```python
from build123d import *

# Parameters (mm, degrees)
SKETCH1_W                      = 19.05
SKETCH1_H                      = 57.15
BOSS_EXTRUDE1_DEPTH            = 25.4
SKETCH8_R                      = 65.0875
CUT_EXTRUDE2_DEPTH             = 89.102674477
SKETCH2_W                      = 17.4625
SKETCH2_H                      = 19.05
SKETCH2_W_2                    = 9.525
CUT_EXTRUDE1_DEPTH             = 43.715256349
CBORE_FOR_M4_SHCS1_D           = 4.5
CBORE_FOR_M4_SHCS1_CBORE_D     = 8
CBORE_FOR_M4_SHCS1_CBORE_DEPTH = 4
SKETCH9_R                      = 3.175
CUT_EXTRUDE3_DEPTH             = 93.307357677
CUT_EXTRUDE4_START             = -6.35
CUT_EXTRUDE4_DEPTH             = 25.4
FILLET1_R                      = 6.35
FILLET2_R                      = 6.35


# Read off the part's stored shape, not the designer's step: Cut-Extrude4
with BuildPart() as part:
    # Sketch1 → Boss-Extrude1 (new body)
    with BuildSketch(Plane(origin=(0, 0, 0), x_dir=(1, 0, 0), z_dir=(0, 1, 0))):
        with Locations((69.85, 0)):
            Rectangle(SKETCH1_W, SKETCH1_H)
    extrude(amount=BOSS_EXTRUDE1_DEPTH)

    # Sketch8 → Cut-Extrude2 (cut, through all)
    with BuildSketch(Plane(origin=(0, 25.4, 0), x_dir=(1, 0, 0), z_dir=(0, 1, 0))):
        Circle(SKETCH8_R)
    extrude(amount=-CUT_EXTRUDE2_DEPTH, mode=Mode.SUBTRACT)

    # Sketch2 → Cut-Extrude1 (cut, through all)
    with BuildSketch(Plane(origin=(79.375, 0, 0), x_dir=(0, 0, -1), z_dir=(1, 0, 0))):
        with Locations((-19.84375, 15.875)):
            Rectangle(SKETCH2_W, SKETCH2_H)
        with Locations((0, 15.875)):
            Rectangle(SKETCH2_W_2, SKETCH2_H)
        with Locations((19.84375, 15.875)):
            Rectangle(SKETCH2_W, SKETCH2_H)
    extrude(amount=-CUT_EXTRUDE1_DEPTH, mode=Mode.SUBTRACT)

    # CBORE for M4 SHCS1 (through all)
    with Locations(Plane(origin=(0, 6.35, 0), x_dir=(1, 0, 0), z_dir=(0, 1, 0))):
        with Locations((69.923370565, -18.735910675), (69.923370565, 18.735910675)):
            CounterBoreHole(CBORE_FOR_M4_SHCS1_D / 2, CBORE_FOR_M4_SHCS1_CBORE_D / 2, CBORE_FOR_M4_SHCS1_CBORE_DEPTH)

    # Sketch9 → Cut-Extrude3 (cut, through all)
    with BuildSketch(Plane.XY.offset(11.1125)):
        with Locations(Location((71.753428179, 19.05, 0), (0, 0, 90))):
            Circle(SKETCH9_R)
    extrude(amount=-CUT_EXTRUDE3_DEPTH, mode=Mode.SUBTRACT)

    # Cut-Extrude4 outline → Cut-Extrude4 (cut)
    with BuildSketch(Plane(origin=(0, 6.35, 0), x_dir=(1, 0, 0), z_dir=(0, 1, 0)).offset(CUT_EXTRUDE4_START)):
        with BuildLine():
            ThreePointArc((74.053089065, 28.575), (78.033180665, 14.533180665), (79.375, 0))
            Line((79.375, 0), (79.375, 28.575))
            Line((79.375, 28.575), (74.053089065, 28.575))
        make_face()
        with BuildLine():
            ThreePointArc((79.375, 0), (78.033180665, -14.533180665), (74.053089065, -28.575))
            Line((74.053089065, -28.575), (79.375, -28.575))
            Line((79.375, -28.575), (79.375, 0))
        make_face()
    extrude(amount=CUT_EXTRUDE4_DEPTH, mode=Mode.SUBTRACT)

    # Fillet1
    fillet1_edges = [part.edges().sort_by_distance(p)[0] for p in [
        (78.976482118, 25.4, 7.943922032),
        (78.976482118, 25.4, -7.943922032),
        (64.600512324, 25.4, 7.947104106),
        (64.600512324, 25.4, -7.947104106),
    ]]
    fillet(fillet1_edges, radius=FILLET1_R)

    # Fillet2
    # the kernel refuses this fillet: 6.35 mm, written as the material it takes off along each edge
    with BuildSketch(Plane(origin=(60.325, -14.878589634, -28.575), x_dir=(1, 0, 0), z_dir=(0, 1, 0))) as fillet2_piece_1:
        with BuildLine():
            CenterArc((5.951435854, -6.35), FILLET2_R, 90, 69.592112093)
            Line((0, -4.135748145), (-0.119028717, -4.091463108))
            ThreePointArc((-0.119028717, -4.091463108), (-0.127, -2.067874072), (-0.127, 0))
            Line((-0.127, 0), (0, 0.127))
            Line((0, 0.127), (5.951435854, 0.127))
            Line((5.951435854, 0.127), (5.951435854, 0))
        make_face()
    extrude(amount=36.107179269, mode=Mode.SUBTRACT)
    with BuildSketch(Plane(origin=(74.053089065, -11.708929515, -28.575), x_dir=(0.33231857215714583, 0, 0.9431671997050343), z_dir=(0, 1, 0))) as fillet2_piece_2:
        with BuildLine():
            CenterArc((4.496228934, -6.347235827), FILLET2_R, 88.309367925, 72.281068131)
            Line((-1.492882784, -4.237012894), (-1.612665019, -4.194808436))
            Line((-1.612665019, -4.194808436), (-0.119782234, 0.042204459))
            Line((-0.119782234, 0.042204459), (-0.003746857, 0.126944717))
            ThreePointArc((-0.003746857, 0.126944717), (2.341785903, 0.161552158), (4.687318663, 0.126944717))
            Line((4.687318663, 0.126944717), (4.683571806, 0))
        make_face()
    extrude(amount=29.76785903, mode=Mode.SUBTRACT)
    with BuildSketch(Plane(origin=(60.325, -14.878589634, 28.575), x_dir=(1, 0, 0), z_dir=(0, 1, 0))) as fillet2_piece_3:
        with BuildLine():
            CenterArc((5.951435854, 6.35), FILLET2_R, 200.407887907, 69.592112093)
            Line((0, 4.135748145), (-0.119028717, 4.091463108))
            ThreePointArc((-0.119028717, 4.091463108), (-0.127, 2.067874072), (-0.127, 0))
            Line((-0.127, 0), (0, -0.127))
            Line((0, -0.127), (5.951435854, -0.127))
            Line((5.951435854, -0.127), (5.951435854, 0))
        make_face()
    extrude(amount=36.107179269, mode=Mode.SUBTRACT)
    with BuildSketch(Plane(origin=(74.053089065, -11.708929515, 28.575), x_dir=(0.3323185721571436, 0, -0.943167199705035), z_dir=(0, 1, 0))) as fillet2_piece_4:
        with BuildLine():
            CenterArc((4.496228934, 6.347235827), FILLET2_R, 199.409563944, 72.281068131)
            Line((-1.492882784, 4.237012894), (-1.612665019, 4.194808436))
            Line((-1.612665019, 4.194808436), (-0.119782234, -0.042204459))
            Line((-0.119782234, -0.042204459), (-0.003746857, -0.126944717))
            ThreePointArc((-0.003746857, -0.126944717), (2.341785903, -0.161552158), (4.687318663, -0.126944717))
            Line((4.687318663, -0.126944717), (4.683571806, 0))
        make_face()
    extrude(amount=29.76785903, mode=Mode.SUBTRACT)


solid = part.part
```
Here's how the part is built. I have some questions about the finished solid (model axes, mm). A direction names the side the tool comes from. Round coordinates to 2 decimals unless told otherwise and drop trailing zeros. Order: outer loops, then holes, each group sorted by start corner. A loop starts at its lowest first (then second) coordinate and runs counter-clockwise, first axis right, second up. Notation, with made-up numbers: (-5, 30.25) -> (25, 30.25) arc R30 ccw to (25, 55.25) -> close; hole circle Ø3 at (38, 69). An arc over 180 degrees is marked (long way). Use a Markdown table: item, result. Add a question column.
(1) For faces 1 (the face through (72, 14, -4.762)), 2 (the face through (71, 14, -11.112)), 3 (the face through (65.5, 6.35, 20)), 4 (the face through (73.739, 4.378, 17.534)), which set-ups out of +Z, -Z, +X, -X, +Y, -Y let a thin tool reach every point of the face, with its end or its side?
(2) Suppose I cut it at C-C, the plane y = 18.5. Count the separate pieces of the cut face and the enclosed holes in it, and give its area (3 significant figures).
(3) I need wall thicknesses on line 1 along Z through (x, y) = (78.25, 8.25); line 2 along Z through (x, y) = (68, 5) (3 decimals); line 3 along Z through (x, y) = (70.5, 5.25). Which ranges of each line are inside material? Lowest first, please.
(4) For pin 1 Ø9 at (x, z) = (68, 18.5) entering from +Y; pin 2 Ø6 at (y, z) = (6, 6.5) entering from +X; pin 3 Ø1.5 at (y, z) = (5.5, 11.5) entering from -X, each with a flat end and sliding along its axis, tell me the tip position at first contact or that it passes through.
(5) Suppose I cut it at B-B, the plane x = 61.75. Please give me the cut outline in (y, z).
(6) If we mould it in two halves opening along X, with no side actions, what happens to faces 5 (the face through (72, 25.4, -8)), 6 (the face through (62.7, 3.13, -27.47)), 7 (the face through (72, 2.35, -17)), 8 (the face through (72.17, 1.16, 18.64))? For each: released by +X, released by -X, zero draft, split by the parting line, or undercut.
Verdict:
| question | item | result |
|---|---|---|
| 1 | face 1 | +X, -X, +Y |
| 1 | face 2 | -Z, +X, -X, +Y |
| 1 | face 3 | +Z, +X, -X, +Y |
| 1 | face 4 | +Y |
| 2 | separate pieces | 4 |
| 2 | enclosed holes | 0 |
| 2 | area | 103 mm2 |
| 3 | line 1 | -11.11 to -4.76, 4.76 to 11.11 |
| 3 | line 2 | -28.575 to -22.243, -15.229 to 15.229, 22.243 to 28.575 |
| 3 | line 3 | -28.51 to -22.69, -14.78 to 14.78, 22.69 to 28.51 |
| 4 | pin 1 | y = 6.35 |
| 4 | pin 2 | x = 79.3 |
| 4 | pin 3 | x = 63.92 |
| 5 | outline | (0, -26.68) -> (6.35, -26.68) -> (6.35, -20.57) -> (0, -20.57) -> close; (0, 20.57) -> (6.35, 20.57) -> (6.35, 26.68) -> (0, 26.68) -> close |
| 6 | face 5 | zero draft |
| 6 | face 6 | released by -X |
| 6 | face 7 | undercut |
| 6 | face 8 | undercut |
